Design review of the part built by this model. Coordinates are the model's own, in mm. A direction names the side the tool comes from. Give positions to 0.01 mm unless a question says otherwise; leave off trailing zeros. Write each loop counter-clockwise with the first axis right and the second up, starting at its lowest first coordinate (ties: lowest second). Pieces come first, ordered by that corner, then holes. Notation, with made-up numbers: M 47,-24.5 L 60,-24.5 A21 cw 60,4.5 Z; hole C 20.5,36 d3. An arc over 180 degrees is marked long. Answer in a Markdown table with one row per item.
Autodesk Inventor part; units mm, degrees
ref_plane "YZ Plane" through (0, 0, 0) normal (1, 0, 0) x (0, 1, 0)
ref_plane "XZ Plane" through (0, 0, 0) normal (0, 1, 0) x (-1, 0, 0)
ref_plane "XY Plane" through (0, 0, 0) normal (0, 0, 1) x (1, 0, 0)
sketch "Sketch1" plane through (0, 0, 0) normal (0, 0, 1) x (1, 0, 0)
  line L0 (-3.25, 35) -> (3.25, 35)
  arc A0 (-13.3333, 3.25) -> (-16, 3.25) centre (-14.6667, 3.25) ccw
  arc A1 (16.0137, 3.25) -> (13.347, 3.25) centre (14.6803, 3.25) ccw
  arc A2 (-3.25, 35) -> (-3.25, 32.3333) centre (-3.25, 33.6667) ccw
  arc A3 (3.25, 32.3333) -> (3.25, 35) centre (3.25, 33.6667) ccw
  line L1 (3.25, 32.3333) -> (3.25, 3.25)
  line L2 (-3.25, 3.25) -> (-3.25, 32.3333)
  line L3 (13.347, 3.25) -> (3.25, 3.25)
  line L4 (-3.25, 3.25) -> (-13.3333, 3.25)
  line L5 (-15.9119, 44.3695) -> (25.0953, 35.2784)
  line L6 (-15.9119, -44.3695) -> (25.0953, -35.2784)
  line L7 (107.2341, 51.0746) -> (107.2341, -58.8764)
  arc A4 (-15.9119, 44.3695) -> (-15.9119, -44.3695) centre (175, 0) ccw
  arc A5 (25.0953, 35.2784) -> (25.0953, -35.2784) centre (175, 0) ccw
  line L8 (-24.8255, 0) -> (30.5939, 0)
  line L9 (-16, 3.25) -> (-16, 0)
  line L10 (16.0137, 3.25) -> (16.0137, 0)
  line L11 (-3.25, -35) -> (3.25, -35)
  arc A6 (-16, -3.25) -> (-13.3333, -3.25) centre (-14.6667, -3.25) ccw
  arc A7 (13.347, -3.25) -> (16.0137, -3.25) centre (14.6803, -3.25) ccw
  arc A8 (-3.25, -32.3333) -> (-3.25, -35) centre (-3.25, -33.6667) ccw
  arc A9 (3.25, -35) -> (3.25, -32.3333) centre (3.25, -33.6667) ccw
  line L12 (3.25, -32.3333) -> (3.25, -3.25)
  line L13 (-3.25, -3.25) -> (-3.25, -32.3333)
  line L14 (13.347, -3.25) -> (3.25, -3.25)
  line L15 (-3.25, -3.25) -> (-13.3333, -3.25)
  line L16 (-16, -3.25) -> (-16, 0)
  line L17 (16.0137, -3.25) -> (16.0137, 0)
  point P0 (0, 0)
  dimension "d3" = 1.3333
  dimension "d4" = 2.6667
  dimension "d14" = 2.6667
  dimension "d15" = 1.3333
  dimension "d26" = 392
  dimension "d30" = 5
  dimension "d38" = 0
  dimension "d40" = 10.097
  dimension "d41" = 0
  dimension "d42" = 3.25
  dimension "d43" = 0
extrude "Extrusion1" add sketch "Sketch1" along normal blind 6 contours A2 L2 L4 A0 L9 L8 A4 L5 A5 L10 A1 L3 L1 A3 L0 | L16 A6 L15 L13 A8 L11 A9 L12 L14 A7 L17 L8 A5 L6 A4
fillet "Fillet1" radius 1.3333 4 edges at (-15.9119, -44.3695, 3) (25.0953, -35.2784, 3) (25.0953, 35.2784, 3) (-15.9119, 44.3695, 3)
properties part number "Feet"
1) Add section C-C (y = -13.5). Write out the cut boundary in (x, z).
Geometry says:
| item | result |
|---|---|
| outline | M -20.53,0 L -3.25,0 L -3.25,6 L -20.53,6 Z; M 3.25,0 L 21.59,0 L 21.59,6 L 3.25,6 Z |
2) Add section B-B (x = -12.5). Write out the cut boundary in (y, z).
Geometry says:
| item | result |
|---|---|
| outline | M -43.61,0 L -3.25,0 L -3.25,6 L -43.61,6 Z; M 3.25,0 L 43.61,0 L 43.61,6 L 3.25,6 Z |
3) Add section A-A (z = 4.75). Write out the cut boundary in (x, y).
Geometry says:
| item | result |
|---|---|
| outline | M -16.21,-43.07 A1.33 ccw -14.62,-44.08 L 23.78,-35.57 A1.33 ccw 24.79,-33.97 A154 cw 24.79,33.97 A1.33 ccw 23.78,35.57 L -14.62,44.08 A1.33 ccw -16.21,43.07 A196 ccw Z; hole M -16,-3.25 A1.33 ccw -13.33,-3.25 L -3.25,-3.25 L -3.25,-32.33 A1.33 ccw -3.25,-35 L 3.25,-35 A1.33 ccw 3.25,-32.33 L 3.25,-3.25 L 13.35,-3.25 A1.33 ccw 16.01,-3.25 L 16.01,3.25 A1.33 ccw 13.35,3.25 L 3.25,3.25 L 3.25,32.33 A1.33 ccw 3.25,35 L -3.25,35 A1.33 ccw -3.25,32.33 L -3.25,3.25 L -13.33,3.25 A1.33 ccw -16,3.25 Z |
4) The part is to be moulded in two halves that separate along Y. For faces 3 (the face through (4.313, 39.886, 2.958)), 4 (the face through (-15.63, -43.9, 3.04)), 5 (the face through (14.651, 4.583, 2.958)), say which applies: released by +Y, released by -Y, zero draft, split by the parting line, or undercut.
Geometry says:
| item | result |
|---|---|
| face 3 | released by +Y |
| face 4 | released by -Y |
| face 5 | undercut |
5) To check wall thickness, follow probe 1 along Y at (x, z) = (-4, 3.4); probe 2 along X at (y, z) = (15.5, 0.6); probe 3 along Y at (x, z) = (-11.5, 2.6). State the ranges of each line that lie inside material, in increasing order. Write a range as [from, to].
Geometry says:
| item | result |
|---|---|
| probe 1 | [-41.73, -34.77], [-32.56, -3.25], [3.25, 32.56], [34.77, 41.73] |
| probe 2 | [-20.39, -3.25], [3.25, 21.78] |
| probe 3 | [-43.39, -3.25], [3.25, 43.39] |
6) Insertion check: P1, Ø1.8, axis at y = -19, z = 4, coming from the +X side; P2, Ø3, axis at y = -15.5, z = 3.5, coming from the -X side; P3, Ø3, axis at y = -28, z = 4, coming from the -X side. Each pin has a flat end and moves straight along its axis. Give the tip position at first contact, or say it passes through.
Geometry says:
| item | result |
|---|---|
| P1 | x = 22.29 |
| P2 | x = -20.5 |
| P3 | x = -19.2 |
7) Add section D-D (y = -38). Write out the cut boundary in (x, z), and give its area (3 significant figures).
Geometry says:
| item | result |
|---|---|
| outline | M -17.28,0 L 12.82,0 L 12.82,6 L -17.28,6 Z |
| area | 181 mm^2 |
8) For faces 1 (the face through (-14.637, -4.583, 2.958)), 2 (the face through (-21, -0.6, 3)), list the 3-axis set-ups (+Z, -Z, +X, -X, +Y, -Y) from which the entire face can be reached by the end or side of a thin tool; tool diameter is ignored.
Geometry says:
| item | result |
|---|---|
| face 1 | +Z, -Z |
| face 2 | +Z, -Z, -X |
